For this review, take the finished solid that the model builds, in its own axes (mm). Face numbers are marked on the shaded views. A direction names the side the tool comes from. Round coordinates to 2 decimals unless told otherwise and drop trailing zeros. Order: outer loops, then holes, each group sorted by start corner. A loop starts at its lowest first (then second) coordinate and runs counter-clockwise, first axis right, second up.
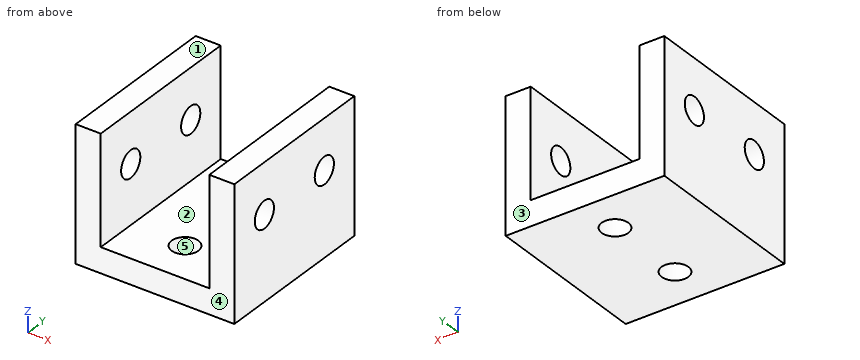
```python
from build123d import *

# Parameters (mm, degrees)
SKETCH_1_W          = 19
SKETCH_1_H          = 20
EXTRUDE_1_DEPTH     = 3
SKETCH_2_W          = 3
SKETCH_2_H          = 20
EXTRUDE_2_DEPTH     = 15
SKETCH_3_R          = 1.6
CUT_EXTRUDE_1_DEPTH = 30
SKETCH_4_R          = 1.6
CUT_EXTRUDE_2_DEPTH = 30
SKETCH_5_W          = 9.97361981
SKETCH_5_H          = 25.467578512
CUT_EXTRUDE_3_DEPTH = 29


with BuildPart() as part:
    # 草图1 → 凸台-拉伸1 (new body)
    with BuildSketch(Plane.XY):
        with Locations((263.488347113, -53.108866795)):
            Rectangle(SKETCH_1_W, SKETCH_1_H)
    extrude(amount=EXTRUDE_1_DEPTH)

    # 草图2 → 凸台-拉伸2 (add)
    with BuildSketch(Plane.XY.offset(3)):
        with Locations((255.488347113, -53.108866795)):
            Rectangle(SKETCH_2_W, SKETCH_2_H)
        with Locations((271.488347113, -53.108866795)):
            Rectangle(SKETCH_2_W, SKETCH_2_H)
    extrude(amount=EXTRUDE_2_DEPTH)

    # 草图3 → 切除-拉伸1 (cut)
    with BuildSketch(Plane.ZY.offset(-253.988347113)):
        with Locations((10, -48.108866795)):
            Circle(SKETCH_3_R)
        with Locations((10, -58.108866795)):
            Circle(SKETCH_3_R)
    extrude(amount=-CUT_EXTRUDE_1_DEPTH, mode=Mode.SUBTRACT)

    # 草图4 → 切除-拉伸2 (cut)
    with BuildSketch(Plane.XY.offset(3)):
        with Locations((263.488347113, -48.108866795)):
            Circle(SKETCH_4_R)
        with Locations((263.488347113, -58.108866795)):
            Circle(SKETCH_4_R)
    extrude(amount=-CUT_EXTRUDE_2_DEPTH, mode=Mode.SUBTRACT)

    # 草图5 → 切除-拉伸3 (cut)
    with BuildSketch(Plane.ZY.offset(-253.988347113)):
        with Locations((20.986809905, -55.842656051)):
            Rectangle(SKETCH_5_W, SKETCH_5_H)
    extrude(amount=-CUT_EXTRUDE_3_DEPTH, mode=Mode.SUBTRACT)


solid = part.part
```
Q1. Take a section at B-B, the plane z = 3.5. State the section outline as (x, y) points, plus the area to 3 significant figures.
Q2. Tool access review of the marked faces 1 and 2: name each direction out of +Z, -Z, +X, -X, +Y, -Y from which nothing blocks a thin tool from reaching the whole face with its end or side.
Q3. Take a section at C-C, the plane y = -47.75. State the section outline as (x, z) points.
Q4. Take a section at D-D, the plane y = -52.5. State the section outline as (x, z) points.
Q5. Mouldability with a two-part tool opening along Y and no side actions: class the marked faces 3, 4 and 5 as +Y half, -Y half, draft (parallel to the pull), parting line (faces both ways), or undercut.
Q6. Wall thickness on line 1 (Y direction, x = 256.35, z = 10); line 2 (X direction, y = -45.25, z = 10); line 3 (X direction, y = -59, z = 2): over which ranges is each line inside the solid? List them lowest first.
Q7. Take a section at A-A, the plane z = 10. State the section outline as (x, y) points.
Q8. Clearance check with a flat-ended pin moving along its axis: pin 1 (4 mm diameter, centred on x = 265.5, y = -56.5, fed in from +Z). State where the tip first meets the part, or that it passes through.
Working result:
1. outline: (253.99, -63.11) - (256.99, -63.11) - (256.99, -43.11) - (253.99, -43.11) - close; (269.99, -63.11) - (272.99, -63.11) - (272.99, -43.11) - (269.99, -43.11) - close
1. area: 120 mm2
2. face 1: +Z, +X, -X, +Y, -Y
2. face 2: +Z, +Y, -Y
3. outline: (253.99, 0) - (261.93, 0) - (261.93, 3) - (256.99, 3) - (256.99, 8.44) - (253.99, 8.44) - close; (253.99, 11.56) - (256.99, 11.56) - (256.99, 16) - (253.99, 16) - close; (265.05, 0) - (272.99, 0) - (272.99, 8.44) - (269.99, 8.44) - (269.99, 3) - (265.05, 3) - close; (269.99, 11.56) - (272.99, 11.56) - (272.99, 16) - (269.99, 16) - close
4. outline: (253.99, 0) - (272.99, 0) - (272.99, 16) - (269.99, 16) - (269.99, 3) - (256.99, 3) - (256.99, 16) - (253.99, 16) - close
5. face 3: +Y half
5. face 4: -Y half
5. face 5: undercut
6. line 1: y = -63.11 to -59.71, -56.51 to -49.71, -46.51 to -43.11
6. line 2: x = 253.99 to 256.99, 269.99 to 272.99
6. line 3: x = 253.99 to 262.16, 264.82 to 272.99
7. outline: (253.99, -63.11) - (256.99, -63.11) - (256.99, -59.71) - (253.99, -59.71) - close; (253.99, -56.51) - (256.99, -56.51) - (256.99, -49.71) - (253.99, -49.71) - close; (253.99, -46.51) - (256.99, -46.51) - (256.99, -43.11) - (253.99, -43.11) - close; (269.99, -63.11) - (272.99, -63.11) - (272.99, -59.71) - (269.99, -59.71) - close; (269.99, -56.51) - (272.99, -56.51) - (272.99, -49.71) - (269.99, -49.71) - close; (269.99, -46.51) - (272.99, -46.51) - (272.99, -43.11) - (269.99, -43.11) - close
8. pin 1: stops at z = 3
